Autodesk Inventor part; units mm, degrees
ref_plane "YZ Plane" through (0, 0, 0) normal (1, 0, 0) x (0, 1, 0)
ref_plane "XZ Plane" through (0, 0, 0) normal (0, 1, 0) x (-1, 0, 0)
ref_plane "XY Plane" through (0, 0, 0) normal (0, 0, 1) x (1, 0, 0)
sketch "Skizze1" plane through (0, 0, 0) normal (0, 1, 0) x (-1, 0, 0)
  line L0 (0, 0) -> (12, 0)
  line L1 (12, 0) -> (12, -16)
  line L2 (12, -16) -> (0, -16)
  line L3 (0, -16) -> (0, 0)
  line L4 (-5, 5) -> (17, 5)
  line L5 (17, 5) -> (17, -21)
  line L6 (17, -21) -> (-5, -21)
  line L7 (-5, -21) -> (-5, 5)
  line L8 (-1, 1) -> (13, 1)
  line L9 (13, 1) -> (13, -17)
  line L10 (13, -17) -> (-1, -17)
  line L11 (-1, -17) -> (-1, 1)
  line L12 (1.75, -1.75) -> (10.25, -1.75)
  line L13 (10.25, -1.75) -> (10.25, -14.25)
  line L14 (10.25, -14.25) -> (1.75, -14.25)
  line L15 (1.75, -14.25) -> (1.75, -1.75)
  line L16 (0.75, -0.75) -> (11.25, -0.75)
  line L17 (11.25, -0.75) -> (11.25, -15.25)
  line L18 (11.25, -15.25) -> (0.75, -15.25)
  line L19 (0.75, -15.25) -> (0.75, -0.75)
  point P0 (6, 0)
  point P1 (6, 5)
  point P2 (6, -16)
  point P3 (12, -8)
  point P4 (6, -1.75)
  point P5 (6, -14.25)
  point P6 (10.25, -8)
  point P7 (1.75, -8)
  dimension "d0" = 16
  dimension "d1" = 12
  dimension "d2" = 5
  dimension "d3" = 5
  dimension "d5" = 5
  dimension "d6" = 5
  dimension "d56" = 1
  dimension "d57" = 1
  dimension "d58" = 1
  dimension "d60" = 1.75
  dimension "d61" = 1.75
  dimension "d63" = 8.5
  dimension "d64" = 1
  dimension "d65" = 1
  dimension "d67" = 1
  dimension "d69" = 12.5
  dimension "d70" = 1
  dimension "d71" = 1.75
  dimension "d72" = 1.75
extrude "Extrusion1" add sketch "Skizze1" along normal blind 1 contours L16 L17 L18 L19
sketch "Skizze2" plane through (0, 0, 0) normal (0, -1, 0) x (1, 0, 0)
  line L0 (21, 19) -> (-33, 19)
  line L1 (-33, 19) -> (-33, -35)
  line L2 (-33, -35) -> (21, -35)
  line L3 (21, -35) -> (21, 19)
  line L4 (-17, -21) -> (-17, 5)
  line L5 (5, -21) -> (-17, -21)
  line L6 (5, 5) -> (5, -21)
  line L7 (-17, 5) -> (5, 5)
  point P0 (0, 0)
  dimension "d11" = 16
  dimension "d12" = 14
  dimension "d13" = 16
  dimension "d14" = 14
  dimension "d35" = 54
  dimension "d36" = 54
extrude "Extrusion2" add sketch "Skizze2" along normal blind 5 contours L3 L2 L1 L0 | L4 L7 L6 L5
sketch "Skizze4" plane through (0, 0, 0) normal (0, 1, 0) x (1, 0, 0)
  line L0 (21, 35) -> (21, -19)
  line L1 (-33, 35) -> (21, 35)
  line L2 (21, -19) -> (-33, -19)
  line L3 (-33, -19) -> (-33, 35)
  point P0 (0, 0)
  point P1 (14, 28)
  point P2 (14, -12)
  point P3 (-26, -12)
  point P4 (-26, 28)
  dimension "d44" = 7
  dimension "d45" = 7
  dimension "d46" = 7
  dimension "d47" = 7
  dimension "d48" = 7
  dimension "d49" = 7
  dimension "d50" = 7
  dimension "d51" = 7
  dimension "d52" = 40
  dimension "d53" = 40
  dimension "d54" = 40
  dimension "d55" = 40
hole "Bohrung1" at (14, 0, -28) at (14, 0, 12) at (-26, 0, 12) at (-26, 0, -28) direction (0, -1, 0) diameter 8.5 depth 5
properties part number "Magazin_1_3D-Druck"
Model file for the job. Use its own axes, mm. Coordinates: 2 decimals unless noted, no trailing zeros. Loops run counter-clockwise (first coordinate to the right, second up) from the corner with the lowest first, then second, coordinate; pieces in that order, holes last. Notation, with made-up numbers: (-18, 14) - (15, 14) arc R25 ccw to (15, 45) - close; hole circle Ø11 at (74.25, 38.25). An arc over 180 degrees is marked (long way). Answer as a JSON object with one key per item and string values. Group by question number.
(1) Cut at D-D (z = -3). Give the cut face in (x, y).
(2) Cut at B-B (z = 12). Give the cut face in (x, y).
(3) Cut at C-C (y = -1.5). Give the cut face in (x, z).
(4) Two-plate mould, pull along Z, no slides. Class faces 1 (the face through (-6, -5, -8)), 2 (the face through (-26.187, -2.535, -32.246)), 3 (the face through (-6, -2, -35)), 4 (the face through (-6, 0, -8)): released by +Z, released by -Z, zero draft, split by the parting line, or undercut.
(5) Cut at A-A (x = -26). Give the cut face in (y, z).
(6) Flat gauge pins, fed straight in: pin 1 (0.8 mm diameter, centred on x = -4.5, y = 0.5, fed in from -Z); pin 2 (2.5 mm diameter, centred on x = -5.5, z = -8, fed in from +Y); pin 3 (0.8 mm diameter, centred on y = 0.5, z = -5, fed in from +X). Where does each tip first touch, or does it go through?
(7) Probe line 1 along Z through (x, y) = (14, -3.8); line 2 along X through (y, z) = (-2.9, -28); line 3 along X through (y, z) = (-3.15, -24.5). List the from-to ranges inside material, lowest first.
Geometry says:
{
 "1": {"outline": "(-33, -5) - (21, -5) - (21, 0) - (-0.75, 0) - (-0.75, 1) - (-1.75, 1) - (-1.75, 0) - (-10.25, 0) - (-10.25, 1) - (-11.25, 1) - (-11.25, 0) - (-33, 0) - close"},
 "2": {"outline": "(-33, -5) - (-30.25, -5) - (-30.25, 0) - (-33, 0) - close; (-21.75, -5) - (9.75, -5) - (9.75, 0) - (-21.75, 0) - close; (18.25, -5) - (21, -5) - (21, 0) - (18.25, 0) - close"},
 "3": {"outline": "(-33, -35) - (21, -35) - (21, 19) - (-33, 19) - close; hole circle Ø8.5 at (-26, -28); hole circle Ø8.5 at (-26, 12); hole circle Ø8.5 at (14, -28); hole circle Ø8.5 at (14, 12)"},
 "4": {"face 1": "zero draft", "face 2": "undercut", "face 3": "released by -Z", "face 4": "undercut"},
 "5": {"outline": "(-5, -35) - (0, -35) - (0, -32.25) - (-5, -32.25) - close; (-5, -23.75) - (0, -23.75) - (0, 7.75) - (-5, 7.75) - close; (-5, 16.25) - (0, 16.25) - (0, 19) - (-5, 19) - close"},
 "6": {"pin 1": "stops at z = -15.25", "pin 2": "stops at y = 0", "pin 3": "stops at x = -0.75"},
 "7": {"line 1": "z = -35 to -32.25, -23.75 to 7.75, 16.25 to 19", "line 2": "x = -33 to -30.25, -21.75 to 9.75, 18.25 to 21", "line 3": "x = -33 to -28.41, -23.59 to 11.59, 16.41 to 21"}
}
